Model file for the job. Use its own axes, mm. Face numbers are marked on the shaded views. A direction names the side the tool comes from. Give positions to 0.01 mm unless a question says otherwise; leave off trailing zeros. Loops run counter-clockwise (first coordinate to the right, second up) from the corner with the lowest first, then second, coordinate; pieces in that order, holes last. Notation, with made-up numbers: (-5.5, 23) -> (25.5, 23) arc R37 ccw to (25.5, 59) -> close; hole circle Ø11 at (54, 49.25). An arc over 180 degrees is marked (long way). Use CSV: the item, a comma, the result in double quotes. Start each with the question number.
(1) Pull direction Z, two halves, no side cores. Call the marked faces 6, 7 and 8: pulls with the +Z half, pulls with the -Z half, needs draft (parallel to the pull), parting line crosses it, or undercut.
(2) Cut at D-D on z = -31. Write the cut outline in (x, y), then the cut area to 3 significant figures.
(3) 3-axis set-ups, long thin cutter, end or side, ignore diameter. For the marked faces 1, 2, 3, 4 and 5: which of +Z, -Z, +X, -X, +Y, -Y reach the whole face in a straight line?
(4) Cut at C-C on y = 5. Write the cut outline in (x, z).
(5) Cut at B-B on z = -79. Write the cut outline in (x, y).
(6) Cut at A-A on x = -49.5. Write the cut outline in (y, z), then the cut area to 3 significant figures.
(7) Drill centre lines: probe 1 along Z at (x, y) = (-4, 0.95); probe 2 along X at (y, z) = (0.8, -15); probe 3 along Z at (x, y) = (-21, 9.5). Where is each one in solid material? Low to high.
(8) Flat gauge pins, fed straight in: pin 1 (3 mm diameter, centred on y = 17.5, z = -33.5, fed in from +X); pin 2 (2 mm diameter, centred on x = -4, z = -15, fed in from -Y) (3 decimals); pin 3 (4 mm diameter, centred on x = -23.5, z = -25.5, fed in from +Y); pin 4 (2.5 mm diameter, centred on x = -26, y = 4.5, fed in from -Z). Where does each tip first touch, or does it go through?
Autodesk Inventor part; units mm, degrees
ref_plane "YZ Plane" through (0, 0, 0) normal (1, 0, 0) x (0, 1, 0)
ref_plane "XZ Plane" through (0, 0, 0) normal (0, 1, 0) x (-1, 0, 0)
ref_plane "XY Plane" through (0, 0, 0) normal (0, 0, 1) x (1, 0, 0)
sketch "Sketch1" plane through (0, 0, 0) normal (0, 1, 0) x (-1, 0, 0)
  line L0 (0, 0) -> (59, 0)
  line L1 (59, 0) -> (59, -91.5)
  line L2 (59, -91.5) -> (0, -91.5)
  line L3 (0, -91.5) -> (0, 0)
  line L4 (4, -15) -> (55, -15) construction
  line L5 (55, -15) -> (55, -79) construction
  line L6 (55, -79) -> (4, -79) construction
  line L7 (4, -79) -> (4, -15) construction
  dimension "d0" = 59
  dimension "d1" = 91.5
  dimension "d2" = 51
  dimension "d3" = 64
  dimension "d4" = 12.5
  dimension "d5" = 4
extrude "Extrusion1" add sketch "Sketch1" along normal blind 1.6
hole "Hole1" at (-55, 0, -15) at (-55, 0, -79) at (-4, 0, -79) at (-4, 0, -15) direction (0, 1, 0) diameter 3.5 end through all
sketch "Sketch2" plane through (0, 1.6, 0) normal (0, 1, 0) x (1, 0, 0)
  circle A0 centre (-49.5, 46) radius 5
  circle A1 centre (-42, 35) radius 5
  line L0 (-59, 0) -> (0, 0)
  line L1 (-59, 91.5) -> (-59, 0)
  line L2 (-52, 0.5) -> (0, 0.5)
  line L3 (0, 0.5) -> (0, 9.5)
  line L4 (0, 9.5) -> (-52, 9.5)
  line L5 (-52, 9.5) -> (-52, 0.5)
  line L6 (-54.5, 82) -> (-2.5, 82)
  line L7 (-2.5, 82) -> (-2.5, 91)
  line L8 (-2.5, 91) -> (-54.5, 91)
  line L9 (-54.5, 91) -> (-54.5, 82)
  line L10 (-9.5, 48) -> (-0.5, 48)
  line L11 (-0.5, 48) -> (-0.5, 60)
  line L12 (-0.5, 60) -> (-9.5, 60)
  line L13 (-9.5, 60) -> (-9.5, 48)
  line L14 (0, 0) -> (0, 91.5)
  dimension "d15" = 10
  dimension "d16" = 10
  dimension "d18" = 46
  dimension "d19" = 9.5
  dimension "d20" = 35
  dimension "d21" = 17
  dimension "d22" = 52
  dimension "d23" = 9
  dimension "d24" = 7
  dimension "d25" = 9.5
  dimension "d26" = 52
  dimension "d27" = 9
  dimension "d28" = 9.5
  dimension "d29" = 4.5
  dimension "d30" = 9
  dimension "d31" = 12
  dimension "d32" = 9.5
  dimension "d33" = 48
extrude "Extrusion2" add sketch "Sketch2" along normal blind 23 contours A0 | A1
extrude "Extrusion3" add sketch "Sketch2" along normal blind 8 contours L5 L4 L3 L2 | L9 L8 L7 L6 | L13 L12 L11 L10
properties part number "Switch Mode PS PCB"
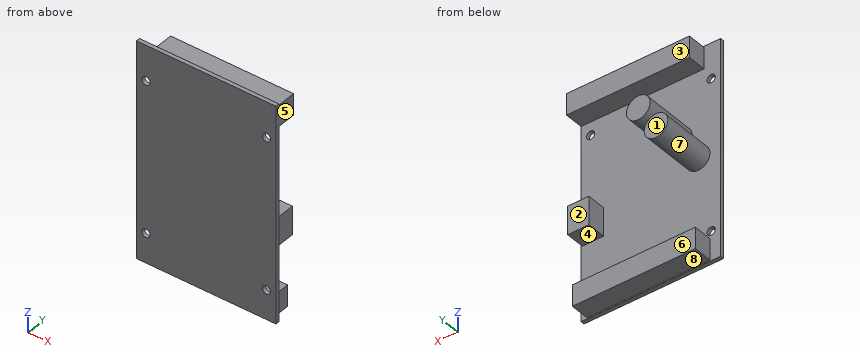
Check result:
1,face 6,"needs draft"
1,face 7,"undercut"
1,face 8,"pulls with the -Z half"
2,outline,"(-59, 0) -> (0, 0) -> (0, 1.6) -> (-39, 1.6) -> (-39, 24.6) -> (-45, 24.6) -> (-45, 1.6) -> (-59, 1.6) -> close"
2,area,"232 mm²"
3,face 1,"+Z, -Z, +X, -X, +Y"
3,face 2,"+Z, -Z, +X, +Y"
3,face 3,"+Z, +X, -X, +Y"
3,face 4,"+X, -X, +Y"
3,face 5,"+Z, -Z, +X, +Y, -Y"
4,outline,"(-54.5, -91) -> (-2.5, -91) -> (-2.5, -82) -> (-54.5, -82) -> close; circle Ø10 at (-49.5, -46); (-52, -9.5) -> (0, -9.5) -> (0, -0.5) -> (-52, -0.5) -> close; circle Ø10 at (-42, -35); (-9.5, -60) -> (-0.5, -60) -> (-0.5, -48) -> (-9.5, -48) -> close"
5,outline,"(-59, 0) -> (-56.75, 0) -> (-56.75, 1.6) -> (-59, 1.6) -> close; (-53.25, 0) -> (-5.75, 0) -> (-5.75, 1.6) -> (-53.25, 1.6) -> close; (-2.25, 0) -> (0, 0) -> (0, 1.6) -> (-2.25, 1.6) -> close"
6,outline,"(0, -91.5) -> (1.6, -91.5) -> (1.6, -91) -> (9.6, -91) -> (9.6, -82) -> (1.6, -82) -> (1.6, -51) -> (24.6, -51) -> (24.6, -41) -> (1.6, -41) -> (1.6, -9.5) -> (9.6, -9.5) -> (9.6, -0.5) -> (1.6, -0.5) -> (1.6, 0) -> (0, 0) -> close"
6,area,"520 mm²"
7,probe 1,"-91.5 to -80.75, -77.25 to -16.75, -13.25 to 0"
7,probe 2,"-59 to -56.75, -53.25 to -5.75, -2.25 to 0"
7,probe 3,"-91 to -82, -9.5 to -0.5"
8,pin 1,"x = -37"
8,pin 2,"through"
8,pin 3,"y = 1.6"
8,pin 4,"z = -91"
